Design review of the part built by this model. Coordinates are the model's own, in mm. Face numbers are marked on the shaded views. A direction names the side the tool comes from. Coordinates: 2 decimals unless noted, no trailing zeros. Loops run counter-clockwise (first coordinate to the right, second up) from the corner with the lowest first, then second, coordinate; pieces in that order, holes last. Notation, with made-up numbers: M 43,-5 L 83,-5 A30 ccw 83,28 Z; hole C 3.25,45.5 d3. An arc over 180 degrees is marked long. Put each result on its own line as item: value. Start each with the question number.
(1) Take a section at A-A, the plane z = 10.5. Give the boundary of the cut face in (x, y), then the cut area to 3 significant figures.
(2) For the marked faces 1 and 2, list the 3-axis set-ups (+Z, -Z, +X, -X, +Y, -Y) from which the entire face can be reached by the end or side of a thin tool; tool diameter is ignored.
(3) The part is to be moulded in two halves that separate along Y. For the marked faces 3, 4 and 5, say which applies: +Y half, -Y half, draft (parallel to the pull), parting line (faces both ways), or undercut.
(4) Take a section at D-D, the plane z = 8. Give the boundary of the cut face in (x, y).
(5) Take a section at C-C, the plane z = 6. Give the boundary of the cut face in (x, y), then the cut area to 3 significant figures.
(6) Take a section at B-B, the plane x = 0. Give the boundary of the cut face in (y, z).
(7) Clearance check with flat-ended pins moving along their axes: pin 1 (6 mm diameter, centred on y = -4, z = 8.5, fed in from +X); pin 2 (0.6 mm diameter, centred on x = 0.5, y = 1.5, fed in from +Z); pin 3 (1.5 mm diameter, centred on x = 0, y = -0.5, fed in from +Z). State where each tip first meets the part, or that it passes through.
(8) For probe 1 along Z at (x, y) = (0.75, 0.25); probe 2 along X at (y, z) = (1, 12.25); probe 3 along Y at (x, z) = (0.5, 10.5), list the stretches that pass through material, from the lowest coordinate up. Write a range as [from, to].
```python
from build123d import *

# Parameters (mm, degrees)
SKETCH1_R           = 5.6
BOSS_EXTRUDE1_DEPTH = 9
SKETCH2_R           = 3.1
BOSS_EXTRUDE2_DEPTH = 3.8
CUT_EXTRUDE1_START  = -0.5
SKETCH3_R           = 1.95
CUT_EXTRUDE1_DEPTH  = 0.5
CHAMFER1_SIZE       = 5
CHAMFER1_SIZE2      = 1.339745962
FILLET1_R           = 2


with BuildPart() as part:
    # Sketch1 → Boss-Extrude1 (new body)
    with BuildSketch(Plane.XY):
        Circle(SKETCH1_R)
    extrude(amount=BOSS_EXTRUDE1_DEPTH)

    # Sketch2 → Boss-Extrude2 (add)
    with BuildSketch(Plane.XY.offset(9)):
        with Locations(Location((0, 0, 0), (0, 0, 180))):
            Circle(SKETCH2_R)
        with BuildLine():
            Line((-1.303840481, -1.45), (1.303840481, -1.45))
            ThreePointArc((1.303840481, -1.45), (1.95, 0), (1.303840481, 1.45))
            Line((1.303840481, 1.45), (-1.303840481, 1.45))
            ThreePointArc((-1.303840481, 1.45), (-1.95, 0), (-1.303840481, -1.45))
        make_face(mode=Mode.SUBTRACT)
    extrude(amount=BOSS_EXTRUDE2_DEPTH)

    # Sketch3 → Cut-Extrude1 (cut)
    with BuildSketch(Plane.XY.offset(12.8).offset(CUT_EXTRUDE1_START)):
        with Locations(Location((0, 0, 0), (0, 0, 131.961888828))):
            Circle(SKETCH3_R)
    extrude(amount=CUT_EXTRUDE1_DEPTH, mode=Mode.SUBTRACT)

    # Chamfer1
    chamfer1_edges = [part.edges().sort_by_distance(p)[0] for p in [
        (-5.6, 0, 9),
    ]]
    chamfer1_side = [part.faces().sort_by_distance(p)[0] for p in [
        (-5.6, 0, 4.5),
    ]]
    chamfer(chamfer1_edges, length=CHAMFER1_SIZE, length2=CHAMFER1_SIZE2, reference=chamfer1_side[0])

    # Fillet1
    # the kernel refuses this fillet: 2 mm, written as the material it takes off along each edge
    with BuildSketch(Plane(origin=(0, 0, 9), x_dir=(1, 0, 0), z_dir=(0, -1, 0))) as fillet1_piece_1:
        with BuildLine():
            CenterArc((2.715609132, -1.962713341), FILLET1_R, 15, 63.919064975)
            Line((3.1, 0), (3.107687817, 0.039254267))
            ThreePointArc((3.107687817, 0.039254267), (3.680127019, 0.04), (4.260254038, 0.04))
            Line((4.260254038, 0.04), (4.298891071, 0.010352762))
            Line((4.298891071, 0.010352762), (4.686097817, -1.434722489))
            Line((4.686097817, -1.434722489), (4.647460784, -1.445075251))
        make_face()
    revolve(axis=Axis((0, 0, 9), (0, 0, 1)), mode=Mode.SUBTRACT)


solid = part.part
```
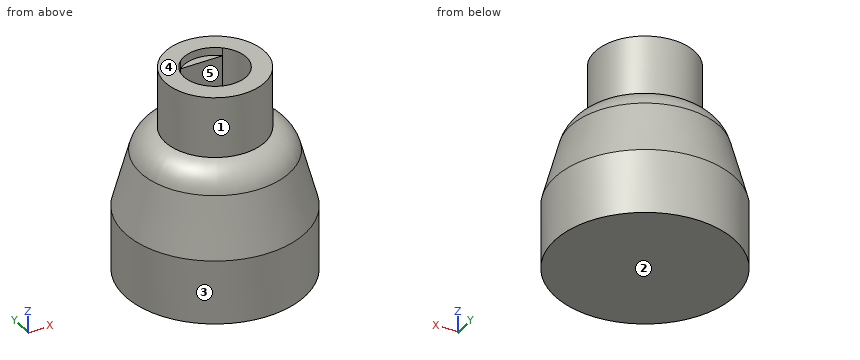
Computed values:
1. outline: C 0,0 d6.2; hole M -1.3,-1.45 L 1.3,-1.45 A1.95 ccw 1.3,1.45 L -1.3,1.45 A1.95 ccw Z
1. area: 20.0 mm^2
2. face 1: +Z
2. face 2: -Z, +X, -X, +Y, -Y
3. face 3: parting line
3. face 4: draft
3. face 5: undercut
4. outline: C 0,0 d8.94
5. outline: C 0,0 d10.13
5. area: 80.6 mm^2
6. outline: M -5.6,0 L 5.6,0 L 5.6,4 L 4.65,7.55 A2 ccw 3.1,9 L 3.1,12.8 L 1.95,12.8 L 1.95,12.3 L 1.45,12.3 L 1.45,9 L -1.45,9 L -1.45,12.3 L -1.95,12.3 L -1.95,12.8 L -3.1,12.8 L -3.1,9 A2 ccw -4.65,7.55 L -5.6,4 Z
7. pin 1: stops at x = 4.61
7. pin 2: stops at z = 12.3
7. pin 3: stops at z = 9
8. probe 1: z = [0, 9]
8. probe 2: x = [-2.93, -1.67], [1.67, 2.93]
8. probe 3: y = [-3.06, -1.45], [1.45, 3.06]
